For this review, use the dimensioned drawing (mm, ordinates from the lowest corner) and the shaded views. Coordinates: 2 decimals unless noted, no trailing zeros. Write each loop counter-clockwise with the first axis right and the second up, starting at its lowest first coordinate (ties: lowest second). Pieces come first, ordered by that corner, then holes. Notation, with made-up numbers: (16.25, 55) - (51.25, 55) arc R23 cw to (51.25, 81) - close; hole circle Ø1 at (43.5, -14.5). An arc over 180 degrees is marked (long way). Answer as a JSON object with one key per item and string values.
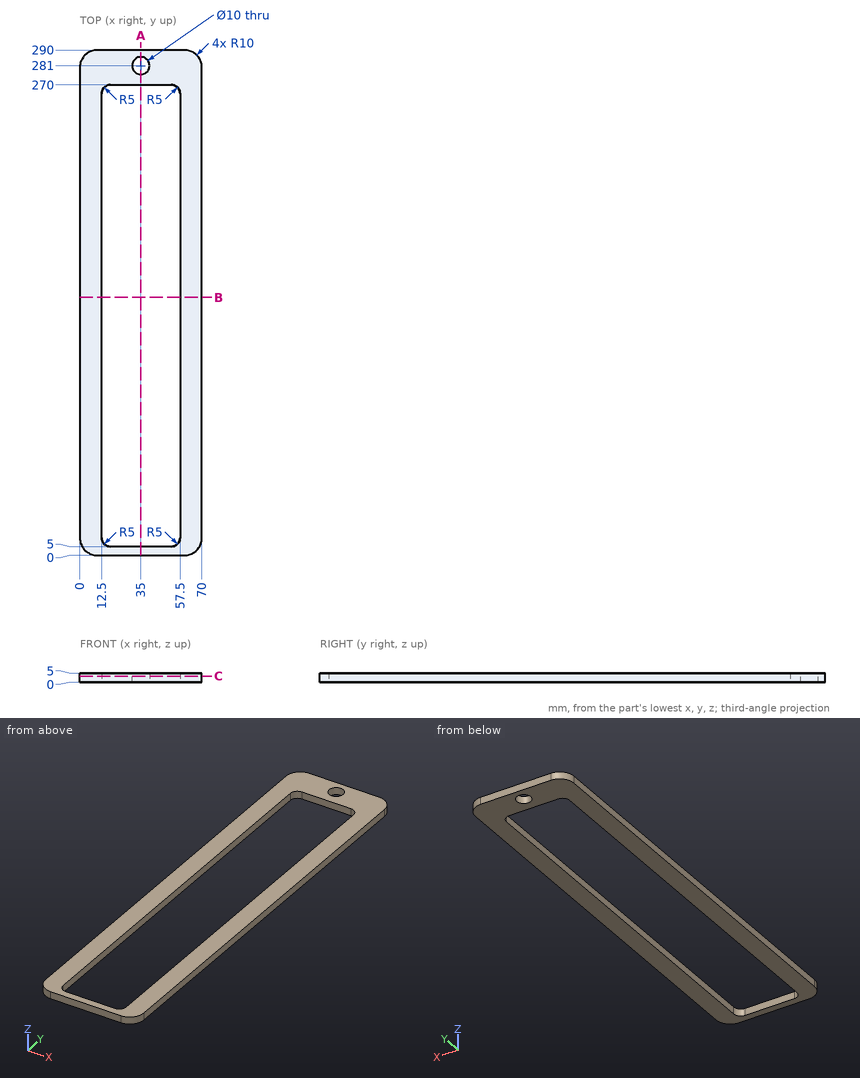
(1) Take a section at C-C, the plane z = 3.35. Write out the cut boundary in (x, y), and give its area (3 significant figures).
Solved:
{"outline": "(0, 10) arc R10 ccw to (10, 0) - (60, 0) arc R10 ccw to (70, 10) - (70, 280) arc R10 ccw to (60, 290) - (10, 290) arc R10 ccw to (0, 280) - close; hole (12.5, 10) arc R5 ccw to (17.5, 5) - (52.5, 5) arc R5 ccw to (57.5, 10) - (57.5, 265) arc R5 ccw to (52.5, 270) - (17.5, 270) arc R5 ccw to (12.5, 265) - close; hole circle Ø10 at (35, 281)", "area": "8,230 mm^2"}
(2) Take a section at A-A, the plane x = 35. Write out the cut boundary in (y, z).
Solved:
{"outline": "(0, 0) - (5, 0) - (5, 5) - (0, 5) - close; (270, 0) - (276, 0) - (276, 5) - (270, 5) - close; (286, 0) - (290, 0) - (290, 5) - (286, 5) - close"}
(3) Take a section at B-B, the plane y = 148. Write out the cut boundary in (x, z), and give its area (3 significant figures).
Solved:
{"outline": "(0, 0) - (12.5, 0) - (12.5, 5) - (0, 5) - close; (57.5, 0) - (70, 0) - (70, 5) - (57.5, 5) - close", "area": "125 mm^2"}
(4) To check wall thickness, follow line 1 (Y direction, x = 35, z = 3.9); line 2 (X direction, y = 146.5, z = 2.6); line 3 (X direction, y = 281, z = 3.05). State the ranges of each line that lie inside material, in increasing order. Write a range as from..to.
Solved:
{"line 1": "y = 0..5, 270..276, 286..290", "line 2": "x = 0..12.5, 57.5..70", "line 3": "x = 0.05..30, 40..69.95"}
(5) For pin 1 (1 mm diameter, centred on x = 7, z = 2, fed in from -Y); pin 2 (1 mm diameter, centred on x = 7.5, z = 2.5, fed in from +Y), all flat-tipped, find the tip position at first contact; note any pin that passes through.
Solved:
{"pin 1": "stops at y = 0.32", "pin 2": "stops at y = 289.8"}
